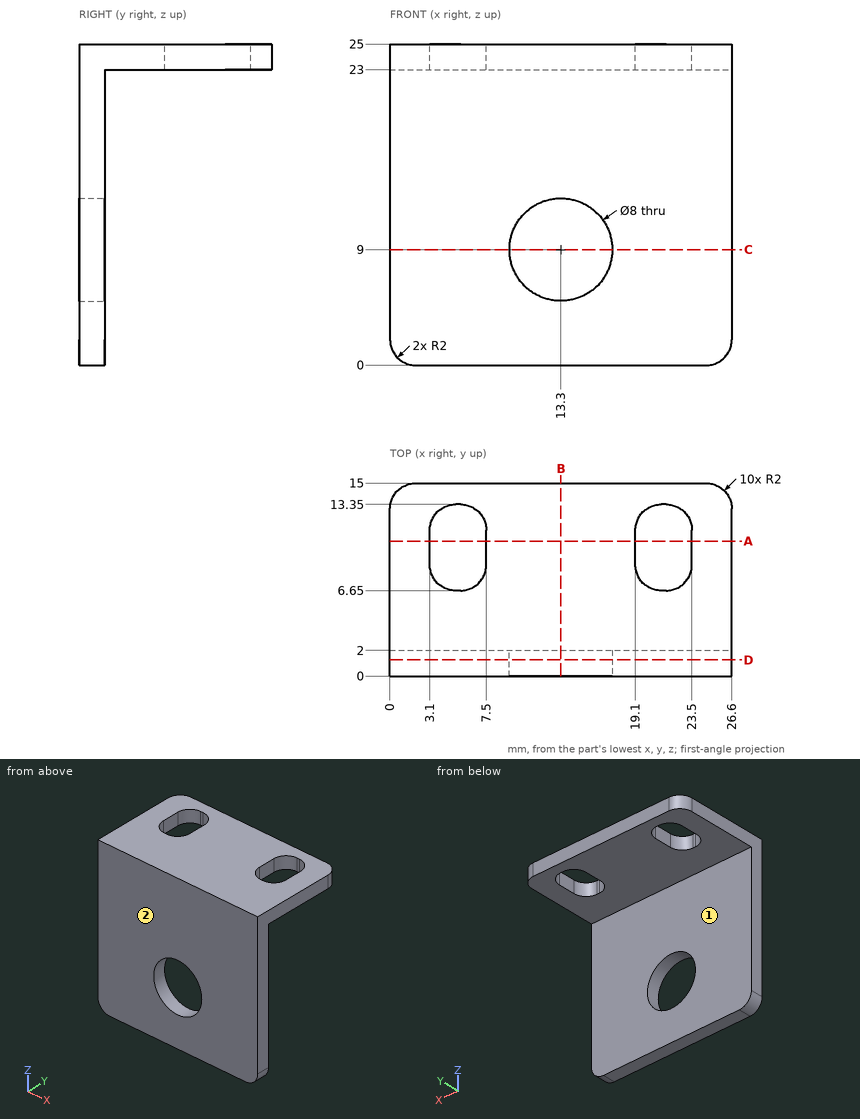
Check sheet for the drawn part. Datum: minimum x, y, z corner. Units: mm. A direction names the side the tool comes from. Round coordinates to 2 decimals unless told otherwise and drop trailing zeros. Order: outer loops, then holes, each group sorted by start corner. A loop starts at its lowest first (then second) coordinate and runs counter-clockwise, first axis right, second up.
1. Section check A-A on y = 10.5. Record the cut outline in (x, z), then the cut area to 3 significant figures.
Final values:
outline: (0, 23) - (3.1, 23) - (3.1, 25) - (0, 25) - close; (7.5, 23) - (19.1, 23) - (19.1, 25) - (7.5, 25) - close; (23.5, 23) - (26.6, 23) - (26.6, 25) - (23.5, 25) - close
area: 35.6 mm2
2. Section check C-C on z = 9. Record the cut outline in (x, y).
Final values:
outline: (0, 0) - (9.3, 0) - (9.3, 2) - (0, 2) - close; (17.3, 0) - (26.6, 0) - (26.6, 2) - (17.3, 2) - close
3. Section check D-D on y = 1.25. Record the cut outline in (x, z).
Final values:
outline: (0, 2) arc R2 ccw to (2, 0) - (24.6, 0) arc R2 ccw to (26.6, 2) - (26.6, 25) - (0, 25) - close; hole circle Ø8 at (13.3, 9)
4. Thickness scan on L1, parallel to Z at x = 13.3, y = 1.2; L2, parallel to X at y = 1.05, z = 9; L3, parallel to Y at x = 7, z = 13.25. Record the ranges inside material, lowest first.
Final values:
L1: z = 0 to 5, 13 to 25
L2: x = 0 to 9.3, 17.3 to 26.6
L3: y = 0 to 2
5. Go/stop test with flat-tipped pins: P1, Ø7, axis at x = 17.5, z = 11.5, coming from the +Y side; P2, Ø4, axis at y = 4.5, z = 14.5, coming from the +X side; P3, Ø2, axis at x = 17, y = 4.5, coming from the -Z side. Record where each tip stops, or that it passes through.
Final values:
P1: stops at y = 2
P2: passes through
P3: stops at z = 23
6. Access from +Z, -Z, +X, -X, +Y, -Y to the whole of each face (thin tool, end or side, straight path). Record for the marked faces 1 and 2.
Final values:
face 1: -Z, +X, -X, +Y
face 2: +Z, -Z, +X, -X, -Y
7. Section check B-B on x = 13.3. Record the cut outline in (y, z).
Final values:
outline: (0, 0) - (2, 0) - (2, 5) - (0, 5) - close; (0, 13) - (2, 13) - (2, 23) - (15, 23) - (15, 25) - (0, 25) - close
